Here's how the part is built. I have some questions about the finished solid (model axes, mm). A direction names the side the tool comes from. Give positions to 0.01 mm unless a question says otherwise; leave off trailing zeros. Write each loop counter-clockwise with the first axis right and the second up, starting at its lowest first coordinate (ties: lowest second). Pieces come first, ordered by that corner, then holes. Notation, with made-up numbers: (-7, 54.5) - (29, 54.5) arc R8 cw to (29, 63.5) - close; hole circle Ø8 at (60.25, 68). An arc over 180 degrees is marked (long way). One line per item, written item: value. Start each with the question number.
1) Imagine slicing it at A-A on y = 41. Write out the boundary of the cut face in (x, z).
2) Imagine slicing it at B-B on x = 39. Write out the boundary of the cut face in (y, z), plus the area to 3 significant figures.
3) We'd pull the mould along X, two halves only. Please class faces 5 (the flat face through (21.5, 8, 1)), 6 (the flat face through (42, 39, 3)), 7 (the cylindrical face through (69.385, 67.043, 1.479)): +X half, -X half, draft (parallel to the pull), parting line (faces both ways), or undercut.
4) Please list where these lines run through material, in increasing order: L1, parallel to X at y = 72, z = 2.3; L2, parallel to X at y = 3.5, z = 1.25; L3, parallel to Y at x = 64.5, z = 0.35. Write a range as [from, to].
5) On a 3-axis mill with a long thin cutter (end or side, diameter ignored), from which of +Z, -Z, +X, -X, +Y, -Y can I reach the whole of each face in a straight line? I mean faces 1 (the flat face through (55, 74, 1)), 2 (the flat face through (57.4, 67, 1)), 3 (the flat face through (42, 39, 0)), 4 (the flat face through (24.5, 1, 1)). Say none if no direction works.
6) I'm going to push flat-ended pins straight in: P1, Ø0.6, axis at x = 58, z = 1, coming from the -Y side; P2, Ø0.9, axis at x = 62, z = 1.5, coming from the +Y side; P3, Ø1.5, axis at y = 1, z = 1, coming from the +X side. Where does each tip first touch, or does it pass through?
from build123d import *

# Parameters (mm, degrees)
BOSS_EXTRUDE1_DEPTH = 3


with BuildPart() as part:
    # Sketch1 → Boss-Extrude1 (new body)
    with BuildSketch(Plane.XY):
        with BuildLine():
            Line((61.5, 71), (65, 71))
            Line((65, 71), (65, 76))
            Line((65, 76), (70, 76))
            Line((70, 76), (70, 71))
            ThreePointArc((70, 71), (69.368032654, 66.988756089), (67.533356838, 63.366129268))
            ThreePointArc((67.533356838, 63.366129268), (48.266790444, 32.772966225), (33, 0))
            Line((33, 0), (33, -5))
            Line((33, -5), (28, -5))
            Line((28, -5), (28, 0))
            Line((28, 0), (24.5, 0))
            Line((24.5, 0), (24.5, 3))
            Line((24.5, 3), (25.6, 3))
            Line((25.6, 3), (25.6, 5.3))
            Line((25.6, 5.3), (24.5, 5.3))
            Line((24.5, 5.3), (24.5, 10))
            Line((24.5, 10), (21.5, 10))
            Line((21.5, 10), (21.5, 5.3))
            Line((21.5, 5.3), (20.4, 5.3))
            Line((20.4, 5.3), (20.4, 3))
            Line((20.4, 3), (21.5, 3))
            Line((21.5, 3), (21.5, 0))
            Line((21.5, 0), (18, 0))
            Line((18, 0), (18, -5))
            Line((18, -5), (13, -5))
            Line((13, -5), (13, 0))
            ThreePointArc((13, 0), (29.165358552, 36.716644135), (50, 71))
            Line((50, 71), (50, 76))
            Line((50, 76), (55, 76))
            Line((55, 76), (55, 71))
            Line((55, 71), (58.5, 71))
            Line((58.5, 71), (58.5, 68))
            Line((58.5, 68), (57.4, 68))
            Line((57.4, 68), (57.4, 65.7))
            Line((57.4, 65.7), (58.5, 65.7))
            Line((58.5, 65.7), (58.5, 61))
            Line((58.5, 61), (61.5, 61))
            Line((61.5, 61), (61.5, 65.7))
            Line((61.5, 65.7), (62.6, 65.7))
            Line((62.6, 65.7), (62.6, 68))
            Line((62.6, 68), (61.5, 68))
            Line((61.5, 68), (61.5, 71))
        make_face()
    extrude(amount=BOSS_EXTRUDE1_DEPTH)


solid = part.part
Numbers:
1. outline: (31.44, 0) - (52.93, 0) - (52.93, 3) - (31.44, 3) - close
2. outline: (14.2, 0) - (54.17, 0) - (54.17, 3) - (14.2, 3) - close
2. area: 120 mm^2
3. face 5: undercut
3. face 6: draft
3. face 7: +X half
4. L1: [50, 55], [65, 70]
4. L2: [14.3, 20.4], [25.6, 34.4]
4. L3: [59.08, 71]
5. face 1: +Z, -Z, +Y
5. face 2: +Z, -Z
5. face 3: -Z, +X, -X, +Y, -Y
5. face 4: +Z, -Z, -Y
6. P1: y = 48.82
6. P2: y = 71
6. P3: x = 33.69
